```python
from build123d import *

# Parameters (mm, degrees)
SKETCH1_W           = 508
SKETCH1_H           = 508
BOSS_EXTRUDE1_DEPTH = 142.24
FILLET1_R           = 76.2
CUT_EXTRUDE1_REACH  = 388.347


with BuildPart() as part:
    # Sketch1 → Boss-Extrude1 (new body)
    with BuildSketch(Plane(origin=(0, 0, 0), x_dir=(1, 0, 0), z_dir=(0, 1, 0))):
        Rectangle(SKETCH1_W, SKETCH1_H)
    extrude(amount=BOSS_EXTRUDE1_DEPTH)

    # Fillet1
    fillet1_edges = [part.edges().sort_by_distance(p)[0] for p in [
        (254, 71.12, 254),
        (-254, 71.12, 254),
        (-254, 71.12, -254),
        (254, 71.12, -254),
    ]]
    fillet(fillet1_edges, radius=FILLET1_R)

    # Sketch2 → Cut-Extrude1 (cut, up to next)
    with BuildSketch(Plane(origin=(0, 142.24, 0), x_dir=(1, 0, 0), z_dir=(0, 1, 0)), mode=Mode.PRIVATE) as cut_extrude1_sk1:
        with BuildLine():
            Line((-241.3, 177.8), (-241.3, -177.8))
            ThreePointArc((-241.3, -177.8), (-222.701280605, -222.701280605), (-177.8, -241.3))
            Line((-177.8, -241.3), (177.8, -241.3))
            ThreePointArc((177.8, -241.3), (222.701280605, -222.701280605), (241.3, -177.8))
            Line((241.3, -177.8), (241.3, 177.8))
            ThreePointArc((241.3, 177.8), (222.701280605, 222.701280605), (177.8, 241.3))
            Line((177.8, 241.3), (-177.8, 241.3))
            ThreePointArc((-177.8, 241.3), (-222.701280605, 222.701280605), (-241.3, 177.8))
        make_face()
    cut_extrude1_tool1 = extrude(cut_extrude1_sk1.sketch, amount=-CUT_EXTRUDE1_REACH, mode=Mode.PRIVATE) & part.part
    add(cut_extrude1_tool1.solids().sort_by_distance((0, 142.24, 0))[0], mode=Mode.SUBTRACT)


solid = part.part
```
Could you check a few things on this model? Use its own coordinates, in mm. A direction names the side the tool comes from. Round coordinates to 2 decimals unless told otherwise and drop trailing zeros. Loops run counter-clockwise (first coordinate to the right, second up) from the corner with the lowest first, then second, coordinate; pieces in that order, holes last. Notation, with made-up numbers: (60, -21) - (92, -21) arc R25 ccw to (92, 15) - close; hole circle Ø7 at (56, -30). An arc over 180 degrees is marked (long way). Answer in a Markdown table with one row per item. Add a question column.
(1) If we section it at C-C (y = 12): Please give me the cut outline in (x, z).
(2) For faces 4 (the face through (-2, 70, -254)), 5 (the face through (222.205, 72.116, 223.192)), which set-ups out of +Z, -Z, +X, -X, +Y, -Y let a thin tool reach every point of the face, with its end or its side?
(3) If we mould it in two halves opening along X, with no side actions, what happens to faces 1 (the face through (-2, 72, 241.3)), 2 (the face through (-232.271, 72.116, -231.086)), 3 (the face through (-2, 70, 254))? For each: pulls with the +X half, pulls with the -X half, needs draft (parallel to the pull), parting line crosses it, or undercut.
(4) If we section it at B-B (x = -97): Please give me the cut outline in (y, z).
(5) If we section it at A-A (z = -135.5): Please give me the cut outline in (x, y), plus the area to 3 significant figures.
(6) I need wall thicknesses on line 1 along X through (y, z) = (107, -4); line 2 along X through (y, z) = (70, 182). Which ranges of each line are inside material? Lowest first, please.
Model answer:
| question | item | result |
|---|---|---|
| 1 | outline | (-254, -177.8) arc R76.2 ccw to (-177.8, -254) - (177.8, -254) arc R76.2 ccw to (254, -177.8) - (254, 177.8) arc R76.2 ccw to (177.8, 254) - (-177.8, 254) arc R76.2 ccw to (-254, 177.8) - close; hole (-241.3, -177.8) arc R63.5 ccw to (-177.8, -241.3) - (177.8, -241.3) arc R63.5 ccw to (241.3, -177.8) - (241.3, 177.8) arc R63.5 ccw to (177.8, 241.3) - (-177.8, 241.3) arc R63.5 ccw to (-241.3, 177.8) - close |
| 2 | face 4 | -Z, +X, -X, +Y, -Y |
| 2 | face 5 | +Y, -Y |
| 3 | face 1 | undercut |
| 3 | face 2 | pulls with the -X half |
| 3 | face 3 | needs draft |
| 4 | outline | (0, -254) - (142.24, -254) - (142.24, -241.3) - (0, -241.3) - close; (0, 241.3) - (142.24, 241.3) - (142.24, 254) - (0, 254) - close |
| 5 | outline | (-254, 0) - (-241.3, 0) - (-241.3, 142.24) - (-254, 142.24) - close; (241.3, 0) - (254, 0) - (254, 142.24) - (241.3, 142.24) - close |
| 5 | area | 3,610 mm² |
| 6 | line 1 | x = -254 to -241.3, 241.3 to 254 |
| 6 | line 2 | x = -253.88 to -241.16, 241.16 to 253.88 |
